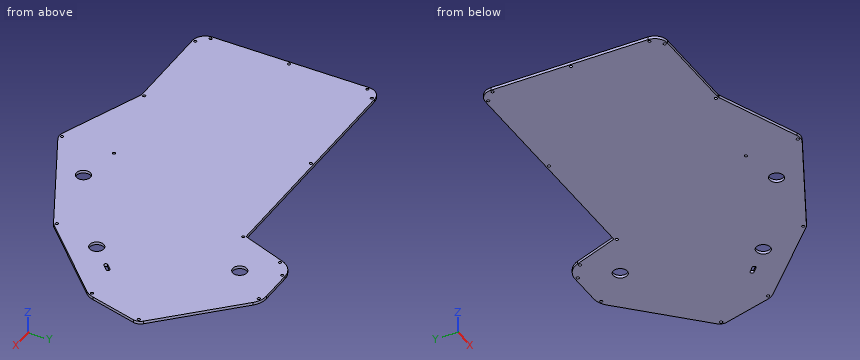
Autodesk Inventor part; units mm, degrees
ref_plane "YZ Plane" through (0, 0, 0) normal (1, 0, 0) x (0, 1, 0)
ref_plane "XZ Plane" through (0, 0, 0) normal (0, 1, 0) x (-1, 0, 0)
ref_plane "XY Plane" through (0, 0, 0) normal (0, 0, 1) x (1, 0, 0)
sketch "Profile" plane through (0, 0, 0) normal (0, 0, 1) x (1, 0, 0)
  arc A0 (-133.951, 77.8406) -> (-145.3411, 66.4505) centre (-133.951, 66.4505) ccw
  line L0 (-133.951, 77.8406) -> (-53.1048, 77.8406)
  line L1 (-34.3215, 77.8406) -> (75.2802, 77.8406)
  line L2 (-53.1048, 77.8406) -> (-34.3215, 77.8406)
  arc A1 (75.2802, 77.8406) -> (76.5082, 78.6945) centre (75.2802, 79.1505) ccw
  line L3 (76.5082, 78.6945) -> (91.3749, 118.7338)
  arc A2 (108.0055, 130.2989) -> (91.3749, 118.7338) centre (108.0055, 112.5588) ccw
  line L4 (108.0055, 130.2989) -> (138.3634, 130.2989)
  arc A3 (150.9075, 125.103) -> (138.3634, 130.2989) centre (138.3634, 112.5588) ccw
  line L5 (150.9075, 125.103) -> (214.354, 61.6565)
  arc A4 (216.4802, 53.7213) -> (214.354, 61.6565) centre (208.545, 55.8476) ccw
  line L6 (216.4802, 53.7213) -> (205.0854, 11.1954)
  arc A5 (200.4939, 3.2427) -> (205.0854, 11.1954) centre (187.9498, 15.7868) ccw
  line L7 (200.4939, 3.2427) -> (135.4341, -61.8171)
  arc A6 (132.5618, -63.9063) -> (135.4341, -61.8171) centre (127.3801, -53.7631) ccw
  line L8 (132.5618, -63.9063) -> (33.0352, -114.7498)
  arc A7 (23.6561, -115.1951) -> (33.0352, -114.7498) centre (27.8535, -104.6066) ccw
  line L9 (23.6561, -115.1951) -> (-50.4135, -85.8326)
  arc A8 (-50.4135, -85.8326) -> (-51.6732, -85.5921) centre (-51.6732, -89.0102) ccw
  line L10 (-51.6732, -85.5921) -> (-133.951, -85.5921)
  arc A9 (-145.3411, -74.202) -> (-133.951, -85.5921) centre (-133.951, -74.202) ccw
  line L11 (-145.3411, -74.202) -> (-145.3411, 66.4505)
  circle A10 centre (-133.951, 75.3205) radius 1.27
  circle A11 centre (-142.8211, 66.4505) radius 1.27
  circle A12 centre (-34.3215, 75.3205) radius 1.27
  circle A13 centre (77.4668, 76.0061) radius 1.27
  circle A14 centre (93.7373, 117.8567) radius 1.27
  circle A15 centre (108.0055, 127.7789) radius 1.27
  circle A16 centre (144.1878, 126.6203) radius 1.27
  circle A17 centre (214.046, 57.3215) radius 1.27
  circle A18 centre (201.1307, 8.1768) radius 1.27
  circle A19 centre (132.5975, -60.9364) radius 1.27
  circle A20 centre (28.2741, -113.4667) radius 1.27
  circle A21 centre (-50.5593, -83.1775) radius 1.27
  circle A22 centre (-133.951, -83.072) radius 1.27
  circle A23 centre (-142.8211, -74.202) radius 1.27
  circle A24 centre (-142.8211, -3.8758) radius 1.27
  line L12 (28.2741, -113.4667) -> (28.2741, -66.8831) construction
  circle A25 centre (28.2741, -66.8831) radius 1.27
  point P0 (0, 0)
  dimension "d2" = 46.5836
extrude "BaseFeature" add sketch "Profile" along normal blind 2.54
sketch "BatteryMount" plane through (0, 0, 2.54) normal (0, 0, 1) x (1, 0, 0)
  circle A0 centre (118.5889, 95.5009) radius 6.35
  circle A1 centre (118.5889, 95.5009) radius 6.35
  arc A2 (102.7139, 117.5989) -> (99.5389, 114.4239) centre (102.7139, 114.4239) ccw
  line L0 (99.5389, 114.4239) -> (99.5389, 76.5779)
  arc A3 (99.5389, 76.5779) -> (102.7139, 73.4029) centre (102.7139, 76.5779) ccw
  line L1 (102.7139, 73.4029) -> (134.4639, 73.4029)
  arc A4 (134.4639, 73.4029) -> (137.6389, 76.5779) centre (134.4639, 76.5779) ccw
  line L2 (137.6389, 76.5779) -> (137.6389, 114.4239)
  arc A5 (137.6389, 114.4239) -> (134.4639, 117.5989) centre (134.4639, 114.4239) ccw
  line L3 (134.4639, 117.5989) -> (102.7139, 117.5989)
  line L4 (138.3634, 130.2989) -> (108.0055, 130.2989)
  point P0 (0, 0)
  dimension "d3" = 37.846
  dimension "d4" = 31.75
  dimension "d5" = 3.175
  dimension "d6" = 12.7
  dimension "d7" = 22.098
  dimension "d8" = 19.05
  dimension "d9" = 12.7
  dimension "d10" = 8.4667
extrude "BatteryMountFeature" cut sketch "BatteryMount" against normal through all contours A0
sketch "Outputs" plane through (0, 0, 2.54) normal (0, 0, 1) x (1, 0, 0)
  circle A0 centre (65.5047, -73.9186) radius 6.35
  circle A1 centre (144.5693, -18.557) radius 6.35
  line L0 (135.4341, -61.8171) -> (200.4939, 3.2427)
  line L1 (33.0352, -114.7498) -> (132.5618, -63.9063) construction
  line L2 (144.5693, -18.557) -> (65.5047, -73.9186) construction
  point P0 (0, 0)
  dimension "d13" = 12.7
  dimension "d14" = 24.13
  dimension "d15" = 21.59
  dimension "d16" = 10
  dimension "d17" = 96.52
extrude "OutputHolesFeature" cut sketch "Outputs" against normal through all
sketch "USB-CInput" plane through (0, 0, 2.54) normal (0, 0, 1) x (1, 0, 0)
  circle A0 centre (162.5298, -0.5965) radius 1.5875
  circle A1 centre (167.0199, 3.8937) radius 1.5875
  line L0 (162.5298, -0.5965) -> (167.0199, 3.8937) construction
  line L1 (135.4341, -61.8171) -> (200.4939, 3.2427) construction
  circle A2 centre (144.5693, -18.557) radius 6.35 construction
  line L2 (162.5298, -0.5965) -> (144.5693, -18.557) construction
  line L3 (161.4072, 0.5261) -> (165.8974, 5.0162)
  line L4 (168.1424, 2.7711) -> (163.6523, -1.719)
  point P0 (0, 0)
  dimension "d20" = 3.175
  dimension "d21" = 25.4
  dimension "d22" = 6.35
extrude "USB-CInputFeature" cut sketch "USB-CInput" against normal through all
properties part number "electronics-cover"
For this review, take the finished solid that the model builds, in its own axes (mm). Round coordinates to 2 decimals unless told otherwise and drop trailing zeros. Loops run counter-clockwise (first coordinate to the right, second up) from the corner with the lowest first, then second, coordinate; pieces in that order, holes last. Notation, with made-up numbers: (52.25, 76.5) - (109.25, 76.5) arc R23 ccw to (109.25, 102.5) - close; hole circle Ø7 at (66, -13). An arc over 180 degrees is marked (long way). One line per item, written item: value. Start each with the question number.
Item 1: For L1, parallel to Y at x = -56, z = 1; L2, parallel to Y at x = 115.5, z = 0.65; L3, parallel to Y at x = 113.5, z = 0.5, list the stretches that pass through material, from the lowest coordinate up.
Item 2: Clearance check with a flat-ended pin moving along its axis: pin 1 Ø1 at (y, z) = (-1.5, 1.5) entering from +X. State where the tip first meets the part, or that it passes through.
Item 3: Take a section at B-B (y = 16.5). Give the boundary of the cut face in (x, z).
Item 4: Take a section at A-A (x = -93). Give the boundary of the cut face in (y, z), plus the area to 3 significant figures.
Item 5: Take a section at C-C (z = 0.8). State how many separate pieces and enclosed holes the cut face has, plus the area to 3 significant figures.
Answer below:
1. L1: y = -85.59 to 77.84
1. L2: y = -72.62 to 89.95, 101.05 to 130.3
1. L3: y = -73.64 to 91.7, 99.3 to 130.3
2. pin 1: stops at x = 196.25
3. outline: (-145.34, 0) - (206.51, 0) - (206.51, 2.54) - (-145.34, 2.54) - close
4. outline: (-85.59, 0) - (77.84, 0) - (77.84, 2.54) - (-85.59, 2.54) - close
4. area: 415 mm2
5. separate pieces: 1
5. enclosed holes: 20
5. area: 59,200 mm2
